Check sheet for the drawn part. Datum: minimum x, y, z corner. Units: mm. A direction names the side the tool comes from. Coordinates: 2 decimals unless noted, no trailing zeros. Write each loop counter-clockwise with the first axis right and the second up, starting at its lowest first coordinate (ties: lowest second). Pieces come first, ordered by that corner, then holes. Notation, with made-up numbers: (72.25, 0) - (122.25, 0) arc R26 ccw to (122.25, 18) - close; hole circle Ø1 at (58.5, 18.25). An arc over 180 degrees is marked (long way). Write each question's results on one line, items separated by ' | '.
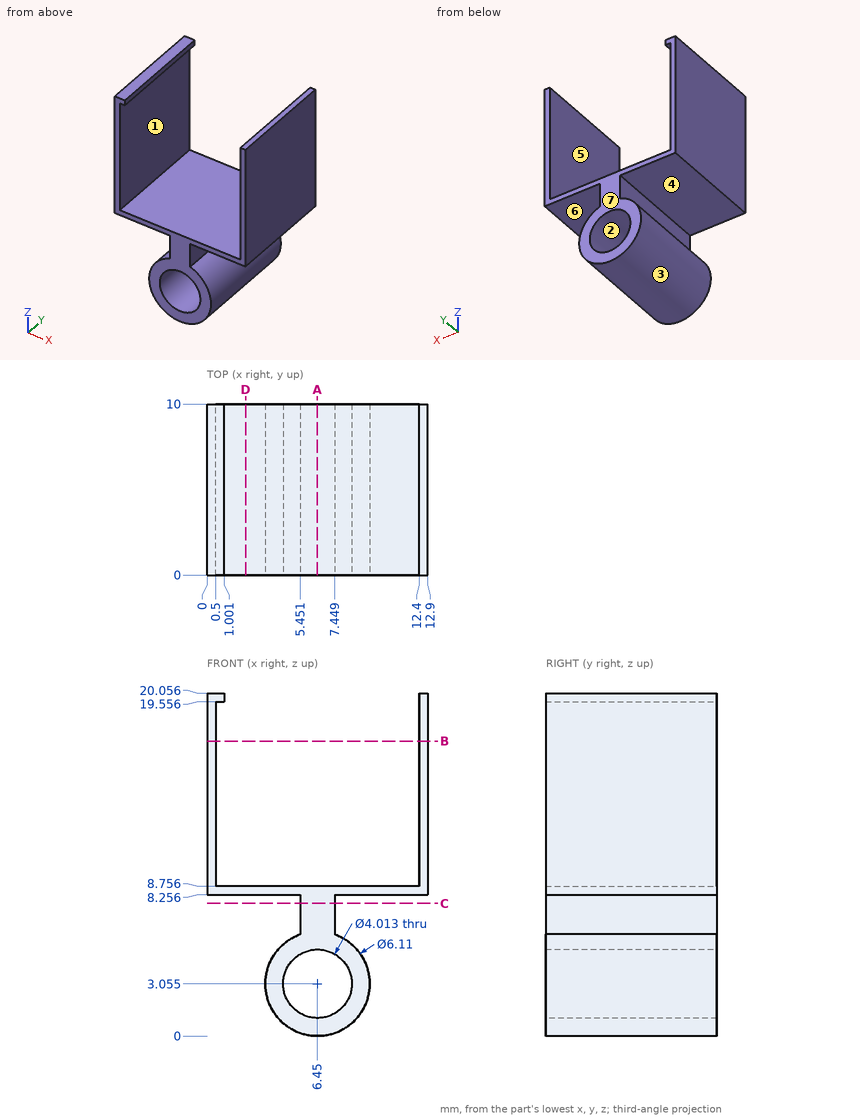
1. Material ranges on L1, parallel to X at y = 8, z = 10; L2, parallel to Z at x = 6.5, y = 6.75; L3, parallel to Z at x = 8.25, y = 8 (1 decimal), recorded low to high. Write a range as [from, to].
Values follow:
L1: x = [0, 0.5], [12.4, 12.9] | L2: z = [0, 1.05], [5.06, 8.76] | L3: z = [0.6, 2.2], [3.9, 5.5], [8.3, 8.8]
2. Draft check along X on the marked faces 1, 2, 3 and 4. Enter one of: pulls with the +X half, pulls with the -X half, needs draft (parallel to the pull), parting line crosses it, or undercut.
Values follow:
face 1: undercut | face 2: undercut | face 3: parting line crosses it | face 4: needs draft
3. Access from +Z, -Z, +X, -X, +Y, -Y to the whole of each face (thin tool, end or side, straight path). Record for the marked faces 5, 6 and 7.
Values follow:
face 5: +Z, +Y, -Y | face 6: +X, +Y, -Y | face 7: +Z, -Z, +X, -X, +Y
4. Sectioned sample at A-A (x = 6.45). Record the cut outline in (y, z).
Values follow:
outline: (0, 0) - (10, 0) - (10, 1.05) - (0, 1.05) - close; (0, 5.06) - (10, 5.06) - (10, 8.76) - (0, 8.76) - close
5. Sectioned sample at D-D (x = 2.25). Record the cut outline in (y, z).
Values follow:
outline: (0, 8.26) - (10, 8.26) - (10, 8.76) - (0, 8.76) - close
6. Sectioned sample at B-B (z = 17.25). Record the cut outline in (x, y), then the cut area to 3 significant figures.
Values follow:
outline: (0, 0) - (0.5, 0) - (0.5, 10) - (0, 10) - close; (12.4, 0) - (12.9, 0) - (12.9, 10) - (12.4, 10) - close | area: 10.0 mm^2
7. Sectioned sample at C-C (z = 7.75). Record the cut outline in (x, y).
Values follow:
outline: (5.45, 0) - (7.45, 0) - (7.45, 10) - (5.45, 10) - close
8. Go/stop test with flat-tipped pins: pin 1 (1.6 mm diameter, centred on x = 10, y = 7, fed in from -Z) (1 decimal); pin 2 (0.7 mm diameter, centred on y = 4.5, z = 7.5, fed in from -X); pin 3 (1.5 mm diameter, centred on x = 11, y = 5, fed in from +Z). Record where each tip stops, or that it passes through.
Values follow:
pin 1: stops at z = 1.7 | pin 2: stops at x = 5.45 | pin 3: stops at z = 8.76
